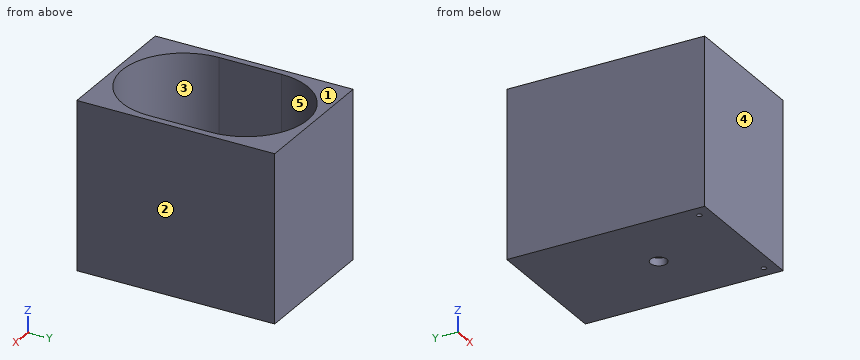
from build123d import *

# Parameters (mm, degrees)
SKETCH4_W                       = 45
SKETCH4_H                       = 65
BOSS_EXTRUDE2_DEPTH             = 55
CUT_EXTRUDE1_DEPTH              = 52.5
F_1_4_28_TAPPED_HOLE1_D         = 5.4102
TAP_DRILL_FOR_M2X0_4_TAP2_D     = 1.6
TAP_DRILL_FOR_M2X0_4_TAP2_DEPTH = 8
TAP_DRILL_FOR_M2X0_4_TAP2_TIP   = 0.480688495
TAP_DRILL_FOR_M2X0_4_TAP3_D     = 1.6
TAP_DRILL_FOR_M2X0_4_TAP3_DEPTH = 8
TAP_DRILL_FOR_M2X0_4_TAP3_TIP   = 0.480688495


with BuildPart() as part:
    # Sketch4 → Boss-Extrude2 (new body)
    with BuildSketch(Plane.XY):
        with Locations((-7.784904398, -11.939291809)):
            Rectangle(SKETCH4_W, SKETCH4_H)
    extrude(amount=BOSS_EXTRUDE2_DEPTH)

    # Sketch5 → Cut-Extrude1 (cut)
    with BuildSketch(Plane.XY.offset(55)):
        with BuildLine():
            Line((-28.034904398, -22.189291809), (-28.034904398, -1.689291809))
            ThreePointArc((-28.034904398, -1.689291809), (-7.784904398, 18.560708191), (12.465095602, -1.689291809))
            Line((12.465095602, -1.689291809), (12.465095602, -22.189291809))
            ThreePointArc((12.465095602, -22.189291809), (-7.784904398, -42.439291809), (-28.034904398, -22.189291809))
        make_face()
    extrude(amount=-CUT_EXTRUDE1_DEPTH, mode=Mode.SUBTRACT)

    # 1/4-28 Tapped Hole1 (through all)
    with Locations(Plane(origin=(0, 0, 0), x_dir=(-1, 0, 0), z_dir=(0, 0, -1))):
        with Locations((7.784904398, -16.439291809)):
            Hole(F_1_4_28_TAPPED_HOLE1_D / 2)

    # Tap Drill for M2x0.4 Tap2
    with Locations(Plane(origin=(0, 0, 0), x_dir=(-1, 0, 0), z_dir=(0, 0, -1))):
        with Locations((-10.715095602, -40.439291809)):
            Hole(TAP_DRILL_FOR_M2X0_4_TAP2_D / 2, depth=TAP_DRILL_FOR_M2X0_4_TAP2_DEPTH)
            with Locations((0, 0, -(TAP_DRILL_FOR_M2X0_4_TAP2_DEPTH + TAP_DRILL_FOR_M2X0_4_TAP2_TIP / 2))):  # 118° drill point
                Cone(0, TAP_DRILL_FOR_M2X0_4_TAP2_D / 2, TAP_DRILL_FOR_M2X0_4_TAP2_TIP, mode=Mode.SUBTRACT)

    # Tap Drill for M2x0.4 Tap3
    with Locations(Plane(origin=(-26.284904398, -40.439291809, 0), x_dir=(-1, 0, 0), z_dir=(0, 0, -1))):
        with Locations((0, 0)):
            Hole(TAP_DRILL_FOR_M2X0_4_TAP3_D / 2, depth=TAP_DRILL_FOR_M2X0_4_TAP3_DEPTH)
            with Locations((0, 0, -(TAP_DRILL_FOR_M2X0_4_TAP3_DEPTH + TAP_DRILL_FOR_M2X0_4_TAP3_TIP / 2))):  # 118° drill point
                Cone(0, TAP_DRILL_FOR_M2X0_4_TAP3_D / 2, TAP_DRILL_FOR_M2X0_4_TAP3_TIP, mode=Mode.SUBTRACT)


solid = part.part
Geometry check sheet. Reference: the model listing, model coordinates, mm. Face numbers are marked on the shaded views. A direction names the side the tool comes from. Round coordinates to 2 decimals unless told otherwise and drop trailing zeros. Loops run counter-clockwise (first coordinate to the right, second up) from the corner with the lowest first, then second, coordinate; pieces in that order, holes last. Notation, with made-up numbers: (33, 0) -> (79, 0) arc R13 cw to (79, 9) -> close; hole circle Ø1 at (-10, -25). An arc over 180 degrees is marked (long way). Answer as a JSON object with one key per item and string values. Group by question number.
Item 1: Release check for a two-part mould opening along X. For the marked faces 1, 2 and 3 record: pulls with the +X half, pulls with the -X half, needs draft (parallel to the pull), parting line crosses it, or undercut.
Item 2: Cross-section at C-C, the plane x = -3.5. Record the cut outline in (y, z), plus the area to 3 significant figures.
Item 3: Cross-section at A-A, the plane y = -15.5. Record the cut outline in (x, z).
Item 4: Cross-section at D-D, the plane z = 5.5. Record the cut outline in (x, y).
Item 5: Set-up check for the marked faces 4 and 5: record each of +Z, -Z, +X, -X, +Y, -Y from which the full face is reachable in a straight line by a thin tool's end or side.
Item 6: Thickness scan on line 1 along X through (y, z) = (-1, 37.5); line 2 along X through (y, z) = (-33.5, 42); line 3 along Y through (x, z) = (-20, 7.5). Record the ranges inside material, lowest first.
Item 7: Depth check by flat-ended pin: pin 1 Ø2 at (x, y) = (-26.28, -40.44) entering from -Z. Enter the tip coordinate at first touch or a pass-through.
Item 8: Cross-section at B-B, the plane z = 44.5. Record the cut outline in (x, y), plus the area to 4 significant figures.
Determined:
{
 "1": {"face 1": "needs draft", "face 2": "pulls with the +X half", "face 3": "undercut"},
 "2": {"outline": "(-44.44, 0) -> (20.56, 0) -> (20.56, 55) -> (18.1, 55) -> (18.1, 2.5) -> (-41.98, 2.5) -> (-41.98, 55) -> (-44.44, 55) -> close", "area": "421 mm²"},
 "3": {"outline": "(-30.28, 0) -> (-10.32, 0) -> (-10.32, 2.5) -> (-28.03, 2.5) -> (-28.03, 55) -> (-30.28, 55) -> close; (-5.25, 0) -> (14.72, 0) -> (14.72, 55) -> (12.47, 55) -> (12.47, 2.5) -> (-5.25, 2.5) -> close"},
 "4": {"outline": "(-30.28, -44.44) -> (14.72, -44.44) -> (14.72, 20.56) -> (-30.28, 20.56) -> close; hole (-28.03, -22.19) arc R20.25 ccw to (12.47, -22.19) -> (12.47, -1.69) arc R20.25 ccw to (-28.03, -1.69) -> close; hole circle Ø1.6 at (-26.28, -40.44); hole circle Ø1.6 at (10.72, -40.44)"},
 "5": {"face 4": "+Z, -Z, +X, -X, -Y", "face 5": "+Z"},
 "6": {"line 1": "x = -30.28 to -28.02, 12.45 to 14.72", "line 2": "x = -30.28 to -24.58, 9.01 to 14.72", "line 3": "y = -44.44 to -38.34, 14.46 to 20.56"},
 "7": {"pin 1": "stops at z = 0"},
 "8": {"outline": "(-30.28, -44.44) -> (14.72, -44.44) -> (14.72, 20.56) -> (-30.28, 20.56) -> close; hole (-28.03, -22.19) arc R20.25 ccw to (12.47, -22.19) -> (12.47, -1.69) arc R20.25 ccw to (-28.03, -1.69) -> close", "area": "806.5 mm²"}
}
